Geometry: final body of the model. Coordinates: model frame, mm. A direction names the side the tool comes from. Give positions to 0.01 mm unless a question says otherwise; leave off trailing zeros. Loops run counter-clockwise (first coordinate to the right, second up) from the corner with the lowest first, then second, coordinate; pieces in that order, holes last.
1. Section B-B, the plane x = 51. Output: boundary loops of the cut face in (y, z), then the cut area to 3 significant figures.
2. First-contact query: P1, Ø3, axis at x = 44.02, y = -26.69, coming from the +Z side; P2, Ø1, axis at y = -81, z = -1.5, coming from the +X side. Flat tips, straight axial feed; report the tip coordinate or a pass-through.
3. Section A-A, the plane y = -44. Output: boundary loops of the cut face in (x, z).
4. Material intervals for line 1 along X through (y, z) = (-83, -2); line 2 along Y through (x, z) = (27, -2.05); line 3 along X through (y, z) = (-82, -1.65), sorted ascending.
5. Section D-D, the plane x = 69.5. Output: boundary loops of the cut face in (y, z), then the cut area to 3 significant figures.
6. Section C-C, the plane z = -2.25. State how many separate pieces and enclosed holes the cut face has, then the cut area to 3 significant figures.
7. Access query for faces 1 (the face through (84.49, -87.44, -1.48)), 2 (the face through (51.42, -46.22, -1.48)). Directions: +Z, -Z, +X, -X, +Y, -Y. A direction counts if a zero-diameter tool reaches every point of the face in a straight line with its end or side. Return the directions, or none.
from build123d import *

# Parameters (mm, degrees)
PAD004_DEPTH    = 3
FILLET016_R     = 6
SKETCH144_R     = 3.75
POCKET031_DEPTH = 5
SKETCH145_R     = 1.75
POCKET058_DEPTH = 3
SKETCH191_R     = 1.65
POCKET060_DEPTH = 3


with BuildPart() as part:
    # Sketch143 → Pad004 (new body)
    with BuildSketch(Plane.XY.offset(45)):
        Polygon((282.000003, 258), (337, 258), (365.924584, 172), (282.000003, 172), align=None)
    extrude(amount=PAD004_DEPTH)

    # Fillet016
    fillet016_edges = [part.edges().sort_by_distance(p)[0] for p in [
        (365.924584, 172, 46.5),
        (282.000003, 172, 46.5),
        (282.000003, 258, 46.5),
        (337, 258, 46.5),
    ]]
    fillet(fillet016_edges, radius=FILLET016_R)

    # Sketch144 (on Face5 of Fillet016) → Pocket031 (cut)
    with BuildSketch(Plane.XY.offset(48)):
        with Locations((302, 230)):
            Circle(SKETCH144_R)
        with Locations((302.000005, 200.000003)):
            Circle(SKETCH144_R)
    extrude(amount=-POCKET031_DEPTH, mode=Mode.SUBTRACT)

    # Sketch145 (on Face5 of Pocket031) → Pocket058 (cut)
    with BuildSketch(Plane.XY.offset(48)):
        with Locations((322.023093, 235.313475)):
            Circle(SKETCH145_R)
        with Locations((334.779262, 196.053817)):
            Circle(SKETCH145_R)
        Polygon((333.263016, 200.720368), (334.214123, 201.029229), (324.489542, 230.958564), (323.538485, 230.649553), (322.587428, 230.340537), (332.311908, 200.411506), align=None)
    extrude(amount=-POCKET058_DEPTH, mode=Mode.SUBTRACT)

    # Sketch191 (on Face5 of Pocket058) → Pocket060 (cut)
    with BuildSketch(Plane.XY.offset(48)):
        with Locations((286.999994, 178.789996)):
            Circle(SKETCH191_R)
        with Locations((287.600004, 252.000004)):
            Circle(SKETCH191_R)
        with Locations((333.100005, 252.500004)):
            Circle(SKETCH191_R)
        with Locations((357, 179)):
            Circle(SKETCH191_R)
    extrude(amount=-POCKET060_DEPTH, mode=Mode.SUBTRACT)


with BuildPart() as part_1:
    # Body015 placement: moved
    add(part.part.moved(Location((0, 0, -2.9))))


with BuildPart() as part_2:
    # Clone placement: moved
    add(part_1.part.moved(Location((-278.000003, -262, -45.1))))


solid = part_2.part
Answers below:
1. outline: (-90, -3) - (-51.4, -3) - (-51.4, 0) - (-90, 0) - close; (-44.92, -3) - (-4, -3) - (-4, 0) - (-44.92, 0) - close
1. area: 239 mm2
2. P1: passes through
2. P2: stops at x = 85.07
3. outline: (4, -3) - (48.6, -3) - (48.6, 0) - (4, 0) - close; (50.7, -3) - (72.45, -3) - (72.45, 0) - (50.7, 0) - close
4. line 1: x = 4 to 7.36, 10.64 to 77.35, 80.65 to 85.49
4. line 2: y = -90 to -64.25, -59.75 to -34.25, -29.75 to -4
4. line 3: x = 4 to 7.88, 10.12 to 77.69, 80.31 to 85.23
5. outline: (-90, -3) - (-35.22, -3) - (-35.22, 0) - (-90, 0) - close
5. area: 164 mm2
6. separate pieces: 1
6. enclosed holes: 9
6. area: 5,730 mm2
7. face 1: +Z, -Z, +X
7. face 2: +Z, -Z
